from build123d import *

# Parameters (mm, degrees)
SKETCH1_R           = 0.75
BOSS_EXTRUDE1_DEPTH = 4
SKETCH3_R           = 2.75
BOSS_EXTRUDE3_DEPTH = 4
SKETCH4_R           = 1.625
CUT_EXTRUDE1_DEPTH  = 4
BOSS_EXTRUDE4_START = 2
SKETCH5_R           = 2.75
SKETCH5_R_2         = 1.625
BOSS_EXTRUDE4_DEPTH = 2


with BuildPart() as part:
    # Sketch1 → Boss-Extrude1 (new body)
    with BuildSketch(Plane(origin=(0, 0, 0), x_dir=(0, 0, -1), z_dir=(1, 0, 0))):
        with BuildLine():
            ThreePointArc((-0.472027972, 1.423794084), (-1.423794084, -0.472027972), (0.472027972, -1.423794084))
            ThreePointArc((0.472027972, -1.423794084), (22.5, 2.132481996), (44.527972028, -1.423794084))
            ThreePointArc((44.527972028, -1.423794084), (46.423794084, -0.472027972), (45.472027972, 1.423794084))
            ThreePointArc((45.472027972, 1.423794084), (22.5, 5.132481996), (-0.472027972, 1.423794084))
        make_face()
        with Locations((45, 0)):
            Circle(SKETCH1_R, mode=Mode.SUBTRACT)
    extrude(amount=BOSS_EXTRUDE1_DEPTH)

    # Sketch3 → Boss-Extrude3 (add)
    with BuildSketch(Plane.ZY):
        Circle(SKETCH3_R)
    extrude(amount=-BOSS_EXTRUDE3_DEPTH)

    # Sketch4 → Cut-Extrude1 (cut)
    with BuildSketch(Plane.ZY):
        Circle(SKETCH4_R)
    extrude(amount=-CUT_EXTRUDE1_DEPTH, mode=Mode.SUBTRACT)

    # Sketch5 → Boss-Extrude4 (add)
    with BuildSketch(Plane.ZY.offset(BOSS_EXTRUDE4_START)):
        Circle(SKETCH5_R)
        Circle(SKETCH5_R_2, mode=Mode.SUBTRACT)
    extrude(amount=-BOSS_EXTRUDE4_DEPTH)


solid = part.part
The listing builds one solid part. Answer for the finished solid, in the listing's coordinates (mm). Coordinates: 2 decimals unless noted, no trailing zeros. Write each loop counter-clockwise with the first axis right and the second up, starting at its lowest first coordinate (ties: lowest second). Pieces come first, ordered by that corner, then holes. Notation, with made-up numbers: M -1.75,40 L 17.25,40 A28 ccw 17.25,71 Z; hole C 26,-6.5 d10. An arc over 180 degrees is marked long. Use one line per item in the form item = value.
Item 1: Given P1, Ø2, axis at y = 0, z = -45, coming from the -X side; P2, Ø1, axis at x = 3, y = -1, coming from the -Z side, each flat-ended and moving along its own axis, determine where each tip first touches the part or whether it passes through.
Model answer:
P1 = 0
P2 = -46.41
Item 2: Find section A-A, the plane z = 0. Give the vertices of the cut face in (x, y) (3 decimals), plus the area to 3 significant figures.
Model answer:
outline = M -2,-2.75 L 4,-2.75 L 4,-1.625 L -2,-1.625 Z; M -2,1.625 L 4,1.625 L 4,2.75 L -2,2.75 Z
area = 13.5 mm2
Item 3: The mould has two halves that part along Z. Classify faces 1 (the face through (1.972, 0.225, -45.715)), 2 (the face through (0, 3, -24)): released by +Z, released by -Z, zero draft, split by the parting line, or undercut.
Model answer:
face_1 = undercut
face_2 = zero draft
Item 4: Find section C-C, the plane x = -1.25. Give the vertices of the cut face in (y, z) (3 decimals), plus the area to 3 significant figures.
Model answer:
outline = C 0,0 d5.5; hole C 0,0 d3.25
area = 15.5 mm2
Item 5: Find section D-D, the plane x = 0.8. Give the vertices of the cut face in (y, z) (3 decimals).
Model answer:
outline = M -1.424,-44.528 A1.5 ccw 1.424,-45.472 A73 ccw 2.121,-1.75 A2.75 ccw long -0.741,-2.648 A70 cw Z; hole C 0,0 d3.25; hole C 0,-45 d1.5
Item 6: Find the intervals of material crossed by probe 1 along Y at (x, z) = (2.25, 0) (3 decimals); probe 2 along X at (y, z) = (4, -32.5); probe 3 along Y at (x, z) = (0.15, -28.5), in increasing order.
Model answer:
probe_1 = -2.75 to -1.625, 1.625 to 2.75
probe_2 = 0 to 4
probe_3 = 1.87 to 4.89
Item 7: Find section B-B, the plane y = 0. Give the vertices of the cut face in (x, z) (3 decimals).
Model answer:
outline = M -2,-2.75 L 0,-2.75 L 0,-5.354 L 4,-5.354 L 4,-1.625 L -2,-1.625 Z; M -2,1.625 L 4,1.625 L 4,2.75 L -2,2.75 Z; M 0,-46.5 L 4,-46.5 L 4,-45.75 L 0,-45.75 Z; M 0,-44.25 L 4,-44.25 L 4,-39.646 L 0,-39.646 Z
